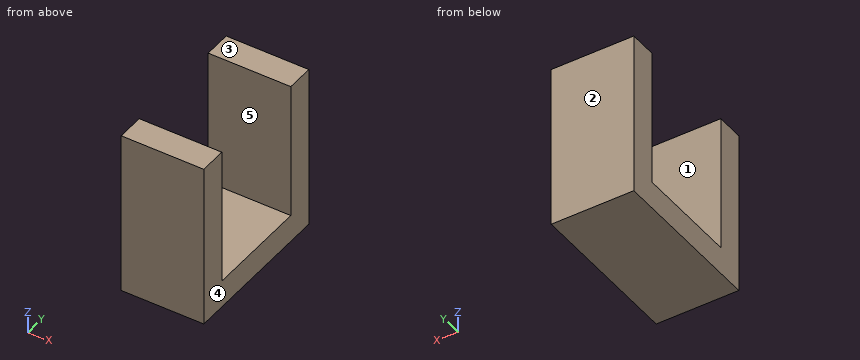
from build123d import *

# Parameters (mm, degrees)
F0_W     = 9
F0_H     = 3
F1_DEPTH = 18
F0_H_2   = 11.5
F2_DEPTH = 3


with BuildPart() as f1:
    # F0 (on Top) → F1 (new body)
    with BuildSketch(Plane.XY):
        with Locations((-37.2173463006, -1.5)):
            Rectangle(F0_W, F0_H)
    extrude(amount=F1_DEPTH)



with BuildPart() as f1b:
    # F0 (on Top) → F1, piece 2 (new body)
    with BuildSketch(Plane.XY):
        with Locations((-37.2173463006, -16)):
            Rectangle(F0_W, F0_H)
    extrude(amount=F1_DEPTH)


with BuildPart() as f1_1:
    add(f1.part)

    add(f1b.part)  # F2 merges F1b
    # F0 (on Top) → F2 (join)
    with BuildSketch(Plane.XY):
        with Locations((-37.2173463006, -8.75)):
            Rectangle(F0_W, F0_H_2)
    extrude(amount=F2_DEPTH)


solid = f1_1.part
Design review of the part built by this model. Coordinates are the model's own, in mm. Face numbers are marked on the shaded views. A direction names the side the tool comes from. Give positions to 0.01 mm unless a question says otherwise; leave off trailing zeros. Loops run counter-clockwise (first coordinate to the right, second up) from the corner with the lowest first, then second, coordinate; pieces in that order, holes last. Notation, with made-up numbers: (29, 81) - (69, 81) arc R15 cw to (69, 101) - close; hole circle Ø6 at (-4.75, -32.5). An arc over 180 degrees is marked (long way). Write item = value, one per line.
1) Take a section at B-B on x = -36. State the section outline as (y, z) points, and give its area (4 significant figures).
Result sheet:
outline = (-17.5, 0) - (0, 0) - (0, 18) - (-3, 18) - (-3, 3) - (-14.5, 3) - (-14.5, 18) - (-17.5, 18) - close
area = 142.5 mm2
2) Draft analysis for pull direction Y (two halves, no side actions). For the marked faces 1, 2 and 3, state which applies: +Y half, -Y half, draft (parallel to the pull), parting line (faces both ways), or undercut.
Result sheet:
face_1 = undercut
face_2 = +Y half
face_3 = draft
3) Take a section at A-A on z = 8. State the section outline as (x, y) points, and give its area (3 significant figures).
Result sheet:
outline = (-41.72, -17.5) - (-32.72, -17.5) - (-32.72, -14.5) - (-41.72, -14.5) - close; (-41.72, -3) - (-32.72, -3) - (-32.72, 0) - (-41.72, 0) - close
area = 54.0 mm2
4) Tool access review of the marked faces 4 and 5: name each direction out of +Z, -Z, +X, -X, +Y, -Y from which nothing blocks a thin tool from reaching the whole face with its end or side.
Result sheet:
face_4 = +Z, -Z, +X, +Y, -Y
face_5 = +Z, +X, -X
5) To check wall thickness, follow line 1 (Y direction, x = -38, z = 7.25); line 2 (Z direction, x = -33.75, y = -4.5). State the ranges of each line that lie inside material, in increasing order.
Result sheet:
line_1 = -17.5 to -14.5, -3 to 0
line_2 = 0 to 3
6) Take a section at C-C on y = -6. State the section outline as (x, z) points, and give its area (3 significant figures).
Result sheet:
outline = (-41.72, 0) - (-32.72, 0) - (-32.72, 3) - (-41.72, 3) - close
area = 27.0 mm2
7) Clearance check with flat-ended pins moving along their axes: pin 1 Ø4.5 at (x, z) = (-37, 14) entering from +Y; pin 2 Ø2.5 at (x, y) = (-35.5, -11.5) entering from +Z. State where each tip first meets the part, or that it passes through.
Result sheet:
pin_1 = 0
pin_2 = 3
